Input: part model. Units: mm. Frame: model coordinates. A direction names the side the tool comes from. Round coordinates to 2 decimals unless told otherwise and drop trailing zeros. Loops run counter-clockwise (first coordinate to the right, second up) from the corner with the lowest first, then second, coordinate; pieces in that order, holes last. Notation, with made-up numbers: (-4.75, -9.5) -> (33.25, -9.5) arc R14 ccw to (33.25, 14.5) -> close; hole circle Ø3 at (39.5, 37.5). An arc over 180 degrees is marked (long way). One line per question, with ' | ' between items. Start each with the question number.
Q1. Access query for faces 1 (the face through (-49.848, 0, 15)), 2 (the face through (49.818, -0.059, 7.212)), 3 (the face through (-56.29, 0.73, 4.95)), 4 (the face through (-45, 0, 25.4)). Directions: +Z, -Z, +X, -X, +Y, -Y. A direction counts if a zero-diameter tool reaches every point of the face in a straight line with its end or side. Return the directions, or none.
Q2. Mould query, pull axis X, two halves, no side actions, for faces 5 (the face through (-1, 3.175, 13)), 6 (the face through (-5.918, 0, 21)), 7 (the face through (-48.604, 0.051, 3.581)). Classes: pulls with the +X half, pulls with the -X half, needs draft (parallel to the pull), parting line crosses it, or undercut.
Q3. Material intervals for L1, parallel to X at y = -3, z = 9; L2, parallel to Z at x = -61, y = 0; L3, parallel to Y at x = -55, z = 3.81 (3 decimals), sorted ascending.
Q4. Cut plane B-B on z = 21. State how many separate pieces and enclosed holes the cut face has, and give its area (3 significant figures).
Q5. Cut plane A-A on z = 11. Return loops of the section in (x, y) (1 decimal).
Q6. Contact query for flat-ended pins moving along their axis: P1, Ø1.9, axis at x = -52.5, y = 1, coming from the +Z side; P2, Ø3, axis at x = 42.5, y = -1, coming from the +Z side; P3, Ø2.5, axis at x = 48.47, y = 0, coming from the -Z side. Output: stop coordinate, or through.
Q7. Cut plane C-C on x = 23. Return loops of the section in (y, z) (3 decimals), and give its area (3 significant figures).
from build123d import *

# Parameters (mm, degrees)
F0_W           = 127
F0_H           = 6.35
F1_DEPTH       = 25.4
F2_W           = 3.81
F2_H           = 19.05
F2_H_2         = 6.35
F3_DEPTH       = 6.35
F4_R           = 1.905
F7_D           = 2.7051
F7_DEPTH       = 14.224
F7_TIP         = 0.8126940303
F7_ON_F6_D     = 2.7051
F7_ON_F6_DEPTH = 14.224
F7_ON_F6_TIP   = 0.8126940303
F8_D           = 2.7051
F8_DEPTH       = 8.89
F8_TIP         = 0.8126940303


with BuildPart() as f1:
    # F0 (on Top) → F1 (new body)
    with BuildSketch(Plane.XY):
        Rectangle(F0_W, F0_H)
    extrude(amount=F1_DEPTH)

    # F2 (on face) → F3 (cut, through all)
    with BuildSketch(Plane.XZ.offset(3.175)):
        with Locations((-51.7525, 15.875)):
            Rectangle(F2_W, F2_H)
        with Locations((-20.0025, 15.875)):
            Rectangle(F2_W, F2_H)
        with Locations((11.7475, 15.875)):
            Rectangle(F2_W, F2_H)
        with Locations((43.4975, 15.875)):
            Rectangle(F2_W, F2_H)
        with Locations((-39.0652, 22.225)):
            Rectangle(F2_W, F2_H_2)
        with Locations((-7.8232, 22.225)):
            Rectangle(F2_W, F2_H_2)
        with Locations((23.4188, 22.225)):
            Rectangle(F2_W, F2_H_2)
        with Locations((54.6608, 22.225)):
            Rectangle(F2_W, F2_H_2)
    extrude(amount=-F3_DEPTH, mode=Mode.SUBTRACT)

    # F4
    f4_edges = [f1.edges().sort_by_distance(p)[0] for p in [
        (-53.6575, 0, 25.4),
        (-49.8475, 0, 25.4),
        (-21.9075, 0, 25.4),
        (-18.0975, 0, 25.4),
        (9.8425, 0, 25.4),
        (13.6525, 0, 25.4),
        (41.5925, 0, 25.4),
        (45.4025, 0, 25.4),
        (-40.9702, 0, 25.4),
        (-37.1602, 0, 25.4),
        (-9.7282, 0, 25.4),
        (-5.9182, 0, 25.4),
        (21.5138, 0, 25.4),
        (25.3238, 0, 25.4),
        (52.7558, 0, 25.4),
        (56.5658, 0, 25.4),
        (63.5, 0, 25.4),
        (-63.5, 0, 25.4),
    ]]
    fillet(f4_edges, radius=F4_R)

    # F7
    with Locations(Plane(origin=(0, 0, 0), x_dir=(1, 0, 0), z_dir=(0, 0, -1))):
        with Locations((-43.2793162763, 0), (48.466347158, 0)):
            Hole(F7_D / 2, depth=F7_DEPTH)
            with Locations((0, 0, -(F7_DEPTH + F7_TIP / 2))):  # 118° drill point
                Cone(0, F7_D / 2, F7_TIP, mode=Mode.SUBTRACT)

    # F7 on F6
    with Locations(Plane(origin=(-63.5, 0, 0), x_dir=(0, -1, 0), z_dir=(-1, 0, 0))):
        with Locations((0, 3.81)):
            Hole(F7_ON_F6_D / 2, depth=F7_ON_F6_DEPTH)
            with Locations((0, 0, -(F7_ON_F6_DEPTH + F7_ON_F6_TIP / 2))):  # 118° drill point
                Cone(0, F7_ON_F6_D / 2, F7_ON_F6_TIP, mode=Mode.SUBTRACT)

    # F8
    with Locations(Plane(origin=(-63.5, 0, 0), x_dir=(0, -1, 0), z_dir=(-1, 0, 0))):
        with Locations((0, 16.51)):
            Hole(F8_D / 2, depth=F8_DEPTH)
            with Locations((0, 0, -(F8_DEPTH + F8_TIP / 2))):  # 118° drill point
                Cone(0, F8_D / 2, F8_TIP, mode=Mode.SUBTRACT)


solid = f1.part
Results:
1) face 1: +Z, +Y, -Y | face 2: -Z | face 3: -X | face 4: +Z, +X, -X, +Y, -Y
2) face 5: needs draft | face 6: undercut | face 7: pulls with the -X half
3) L1: -63.5 to -53.66, -49.85 to -21.91, -18.1 to 9.84, 13.65 to 41.59, 45.4 to 63.5 | L2: 0 to 2.46, 5.16 to 15.16, 17.86 to 25.4 | L3: -3.175 to -1.353, 1.353 to 3.175
4) separate pieces: 9 | enclosed holes: 0 | area: 613 mm^2
5) outline: (-63.5, -3.2) -> (-53.7, -3.2) -> (-53.7, 3.2) -> (-63.5, 3.2) -> close; (-49.8, -3.2) -> (-21.9, -3.2) -> (-21.9, 3.2) -> (-49.8, 3.2) -> close; (-18.1, -3.2) -> (9.8, -3.2) -> (9.8, 3.2) -> (-18.1, 3.2) -> close; (13.7, -3.2) -> (41.6, -3.2) -> (41.6, 3.2) -> (13.7, 3.2) -> close; (45.4, -3.2) -> (63.5, -3.2) -> (63.5, 3.2) -> (45.4, 3.2) -> close; hole circle Ø2.7 at (-43.3, 0); hole circle Ø2.7 at (48.5, 0)
6) P1: z = 6.35 | P2: z = 24.88 | P3: z = 14.28
7) outline: (-3.175, 0) -> (3.175, 0) -> (3.175, 19.05) -> (-3.175, 19.05) -> close | area: 121 mm^2
